Autodesk Inventor part; units mm, degrees
ref_plane "YZ Plane" through (0, 0, 0) normal (1, 0, 0) x (0, 1, 0)
ref_plane "XZ Plane" through (0, 0, 0) normal (0, 1, 0) x (-1, 0, 0)
ref_plane "XY Plane" through (0, 0, 0) normal (0, 0, 1) x (1, 0, 0)
sketch "Sketch1" plane through (0, 0, 0) normal (0, 0, 1) x (1, 0, 0)
  line L0 (-45, 57.5) -> (45, 57.5)
  line L1 (45, 57.5) -> (45, -57.5)
  line L2 (45, -57.5) -> (-45, -57.5)
  line L3 (-45, -57.5) -> (-45, 57.5)
  line L4 (-45, 57.5) -> (45, -57.5) construction
  line L5 (45, 57.5) -> (-45, -57.5) construction
  point P0 (0, 0)
  dimension "d0" = 90
  dimension "d1" = 115
extrude "Extrusion1" add sketch "Sketch1" along normal mid plane 10
sketch "Sketch2" plane through (45, -57.5, 5) normal (1, 0, 0) x (0, 0, -1)
  line L0 (10, 0) -> (0, 0)
  line L1 (10, 115) -> (10, 0)
  point P0 (5, 57.5)
  point P1 (5, 20)
  point P2 (5, 57.5)
  point P3 (5, 95)
  dimension "d4" = 20
  dimension "d5" = 5
  dimension "d8" = 37.5
hole "Hole1" at (45, -37.5, 0) at (45, 0, 0) at (45, 37.5, 0) direction (-1, 0, 0) diameter 3.175 depth 5
sketch "Sketch3" plane through (-45, -57.5, 5) normal (0, -1, 0) x (1, 0, 0)
  line L0 (0, 0) -> (0, -10)
  line L1 (90, -10) -> (0, -10)
  point P0 (45, -5)
  point P1 (25, -5)
  point P2 (75, -5)
  dimension "d20" = 25
  dimension "d21" = 5
  dimension "d24" = 50
hole "Hole2" at (-20, -57.5, 0) at (30, -57.5, 0) direction (0, 1, 0) diameter 3.175 depth 5
sketch "Sketch4" plane through (-45, 57.5, 5) normal (0, 1, 0) x (1, 0, 0)
  line L0 (0, 10) -> (0, 0)
  line L1 (90, 0) -> (0, 0)
  point P0 (45, 5)
  point P1 (25, 5)
  point P2 (75, 5)
  dimension "d36" = 25
  dimension "d37" = 5
  dimension "d40" = 50
hole "Hole3" at (-20, 57.5, 0) at (30, 57.5, 0) direction (0, -1, 0) diameter 3.175 depth 5
sketch "Sketch5" plane through (0, 0, 5) normal (0, 0, 1) x (1, 0, 0)
  line L0 (-45, 57.5) -> (-45, -57.5)
  line L1 (-45, -57.5) -> (45, -57.5)
  point P0 (0, 0)
  point P1 (-40, -37.5)
  point P2 (-40, 0)
  point P3 (-40, 37.5)
  dimension "d52" = 5
  dimension "d53" = 20
  dimension "d56" = 37.5
hole "Hole4" at (-40, -37.5, 5) at (-40, 0, 5) at (-40, 37.5, 5) direction (0, 0, -1) diameter 3.175 depth 5
sketch "Sketch6" plane through (0, 0, 5) normal (0, 0, 1) x (1, 0, 0)
  line L0 (40, -52.5) -> (-35, -52.5)
  line L1 (-35, -52.5) -> (-35, 52.5)
  line L2 (-35, 52.5) -> (40, 52.5)
  line L3 (40, 52.5) -> (40, -52.5)
  line L4 (40, -52.5) -> (-35, 52.5) construction
  line L5 (-35, -52.5) -> (40, 52.5) construction
  line L6 (-45, 57.5) -> (-45, -57.5)
  line L7 (45, 57.5) -> (-45, 57.5)
  line L8 (45, -57.5) -> (45, 57.5)
  line L9 (-45, -57.5) -> (45, -57.5)
  point P0 (0, 0)
  point P1 (2.5, 0)
  dimension "d68" = 10
  dimension "d69" = 5
  dimension "d72" = 5
  dimension "d74" = 5
extrude "Extrusion2" cut sketch "Sketch6" against normal blind 7 contours L0 L1 L2 L3
sketch "Sketch7" plane through (0, 0, -2) normal (0, 0, 1) x (1, 0, 0)
  line L0 (35, -47.5) -> (-30, -47.5)
  line L1 (-30, -47.5) -> (-30, 47.5)
  line L2 (-30, 47.5) -> (35, 47.5)
  line L3 (35, 47.5) -> (35, -47.5)
  line L4 (35, -47.5) -> (-30, 47.5) construction
  line L5 (-30, -47.5) -> (35, 47.5) construction
  line L6 (40, 52.5) -> (40, -52.5)
  line L7 (-35, -52.5) -> (-35, 52.5)
  line L8 (-35, 52.5) -> (40, 52.5)
  line L9 (40, -52.5) -> (-35, -52.5)
  point P0 (0, 0)
  point P1 (2.5, 0)
  dimension "d77" = 5
  dimension "d78" = 5
  dimension "d79" = 5
  dimension "d81" = 5
extrude "Extrusion3" cut sketch "Sketch7" against normal through all contours L0 L1 L2 L3
properties part number "leftright"
Model file for the job. Use its own axes, mm. A direction names the side the tool comes from. Give positions to 0.01 mm unless a question says otherwise; leave off trailing zeros. Order: outer loops, then holes, each group sorted by start corner. A loop starts at its lowest first (then second) coordinate and runs counter-clockwise, first axis right, second up. Notation, with made-up numbers: (72.5, -5.5) -> (115.5, -5.5) arc R26 cw to (115.5, 32.5) -> close; hole circle Ø11 at (24.5, 26). An arc over 180 degrees is marked (long way). Use CSV: the item, a comma, the result in double quotes.
1. 3-axis set-ups, long thin cutter, end or side, ignore diameter. For faces 1 (the flat face through (3, -47.5, -3)), 2 (the cylindrical face through (42.465, 35.926, 0.207)), 3 (the flat face through (2, 52.5, 2)): which of +Z, -Z, +X, -X, +Y, -Y reach the whole face in a straight line?
Outcome:
face 1,"+Z, -Z"
face 2,"+X"
face 3,"+Z"
2. Band-saw the part on D-D, the plane z = -3.25. Give the cut face in (x, y), then the cut area to 4 significant figures.
Outcome:
outline,"(-45, -57.5) -> (45, -57.5) -> (45, 57.5) -> (-45, 57.5) -> close; hole (-30, -47.5) -> (35, -47.5) -> (35, 47.5) -> (-30, 47.5) -> close"
area,"4,175 mm²"
3. Mould opens along Z. For faces 4 (the flat face through (-40, 0, 0)), 5 (the cylindrical face through (-18.45, -54.96, 0.34)), 6 (the cylindrical face through (-18.45, 54.96, -0.34)), 7 (the flat face through (45, 1, -2)) say: +Z half, -Z half, draft (parallel to the pull), parting line (faces both ways), or undercut.
Outcome:
face 4,"+Z half"
face 5,"undercut"
face 6,"undercut"
face 7,"draft"
4. Band-saw the part on C-C, the plane x = 8. Give the cut face in (y, z).
Outcome:
outline,"(-57.5, -5) -> (-47.5, -5) -> (-47.5, -2) -> (-52.5, -2) -> (-52.5, 5) -> (-57.5, 5) -> close; (47.5, -5) -> (57.5, -5) -> (57.5, 5) -> (52.5, 5) -> (52.5, -2) -> (47.5, -2) -> close"
5. Band-saw the part on B-B, the plane y = 43. Give the cut face in (x, z), then the cut area to 3 significant figures.
Outcome:
outline,"(-45, -5) -> (-30, -5) -> (-30, -2) -> (-35, -2) -> (-35, 5) -> (-45, 5) -> close; (35, -5) -> (45, -5) -> (45, 5) -> (40, 5) -> (40, -2) -> (35, -2) -> close"
area,"180 mm²"
6. Drop flat-ended pins along their axis: pin 1 (3.5 mm diameter, centred on y = 37.5, z = 0, fed in from +X); pin 2 (2.5 mm diameter, centred on x = -40, y = 0, fed in from +Z); pin 3 (2.5 mm diameter, centred on y = -37.5, z = 0, fed in from +X). Give the stop position or say it passes through.
Outcome:
pin 1,"x = 45"
pin 2,"z = 0"
pin 3,"x = -35"
7. Band-saw the part on A-A, the plane x = -20. Give the cut face in (y, z), then the cut area to 4 significant figures.
Outcome:
outline,"(-57.5, -5) -> (-47.5, -5) -> (-47.5, -2) -> (-52.5, -2) -> (-52.5, -1.59) -> (-57.5, -1.59) -> close; (-57.5, 1.59) -> (-52.5, 1.59) -> (-52.5, 5) -> (-57.5, 5) -> close; (47.5, -5) -> (57.5, -5) -> (57.5, -1.59) -> (52.5, -1.59) -> (52.5, -2) -> (47.5, -2) -> close; (52.5, 1.59) -> (57.5, 1.59) -> (57.5, 5) -> (52.5, 5) -> close"
area,"98.25 mm²"
8. Drill centre lines: line 1 along Y through (x, z) = (-40, 3.75); line 2 along X through (y, z) = (53.6, 0); line 3 along X through (y, z) = (27, -1.25). Where is each one in solid material? Low to high. Write a range as from..to.
Outcome:
line 1,"-57.5..-39.09, -35.91..-1.59, 1.59..35.91, 39.09..57.5"
line 2,"-45..-21.59, -18.41..28.41, 31.59..45"
line 3,"-45..-35, 40..45"
